Here's how the part is built. I have some questions about the finished solid (model axes, mm). Give positions to 0.01 mm unless a question says otherwise; leave off trailing zeros. Order: outer loops, then holes, each group sorted by start corner. A loop starts at its lowest first (then second) coordinate and runs counter-clockwise, first axis right, second up. Notation, with made-up numbers: M -31,-12.75 L -11,-12.75 A22 cw -11,25.25 Z; hole C -12.75,83 d7. An arc over 180 degrees is marked long. One line per item, written item: value. Start each with the question number.
from build123d import *

# Parameters (mm, degrees)
BOSS_EXTRUDE1_DEPTH = 3
FILLET1_R           = 4
FILLET2_R           = 3
FILLET3_R           = 1
FILLET4_R           = 0.5
SKETCH2_R           = 1
CUT_EXTRUDE1_DEPTH  = 2.3


with BuildPart() as part:
    # Sketch1 → Boss-Extrude1 (new body)
    with BuildSketch(Plane(origin=(0, 0, 0), x_dir=(1, 0, 0), z_dir=(0, 1, 0))):
        with BuildLine():
            Line((8.991433994, -0.392574486), (11.957374237, 67.538625463))
            ThreePointArc((11.957374237, 67.538625463), (7.303664413, 76.769797523), (-2.998880838, 77.623679297))
            Line((-2.998880838, 77.623679297), (-2.998880838, 43.087780912))
            Line((-2.998880838, 43.087780912), (-8.998880838, 39.623679297))
            Line((-8.998880838, 39.623679297), (-8.998880838, -0.141928385))
            ThreePointArc((-8.998880838, -0.141928385), (-0.125378351, -8.999126639), (8.991433994, -0.392574486))
        make_face()
    extrude(amount=BOSS_EXTRUDE1_DEPTH)

    # Fillet1
    fillet1_edges = [part.edges().sort_by_distance(p)[0] for p in [
        (-2.998880838, 1.5, -43.087780912),
    ]]
    fillet(fillet1_edges, radius=FILLET1_R)

    # Fillet2
    fillet2_edges = [part.edges().sort_by_distance(p)[0] for p in [
        (-2.998880838, 1.5, -77.623679297),
    ]]
    fillet(fillet2_edges, radius=FILLET2_R)

    # Fillet3
    fillet3_edges = [part.edges().sort_by_distance(p)[0] for p in [
        (-8.998880838, 1.5, -39.623679297),
    ]]
    fillet(fillet3_edges, radius=FILLET3_R)

    # Fillet4
    fillet4_edges = [part.edges().sort_by_distance(p)[0] for p in [
        (10.474404116, 3, -33.573025488),
        (-0.125378351, 3, 8.999126639),
        (-8.998880838, 3, -19.452200321),
        (-2.998880838, 3, -60.423029196),
        (-3.534779223, 3, -43.397181989),
        (8.325091375, 3, -75.986589378),
        (-2.306460594, 3, -77.365925089),
        (-6.748880838, 3, -40.922717403),
        (-8.864906242, 3, -39.546329028),
    ]]
    fillet(fillet4_edges, radius=FILLET4_R)

    # Sketch2 → Cut-Extrude1 (cut)
    with BuildSketch(Plane(origin=(0, 0, 0), x_dir=(-1, 0, 0), z_dir=(0, -1, 0))):
        with Locations((-6.916463595, 69.482266802)):
            Circle(SKETCH2_R)
        with Locations((-2.740849282, 1.610591965)):
            Circle(SKETCH2_R)
        with Locations((6, 35.355339106)):
            Circle(SKETCH2_R)
    extrude(amount=-CUT_EXTRUDE1_DEPTH, mode=Mode.SUBTRACT)


solid = part.part
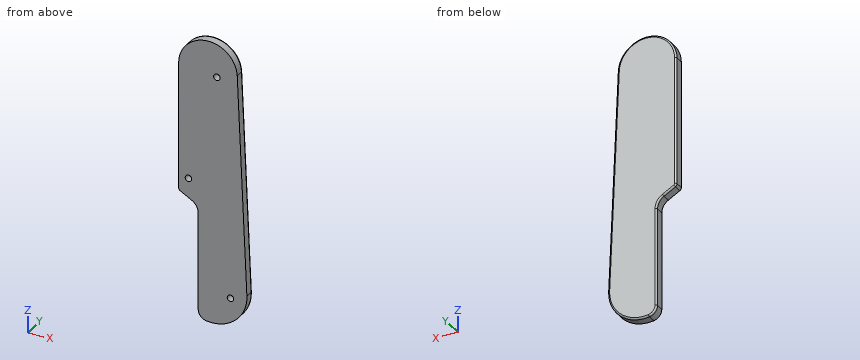
Item 1: I want a section at A-A on y = 0.95. Write out the boundary of the cut face in (x, z), plus the area to 3 significant figures.
Item 2: Will these pins go through, and if not, where does the flat tip stop? P1, Ø1.2, axis at x = -6, z = -35.36, coming from the -Y side; P2, Ø1, axis at y = 2, z = -10, coming from the +X side.
Item 3: Please list where these lines run through material, in increasing order: probe 1 along X at (y, z) = (0.45, -35); probe 2 along Z at (x, y) = (-6, 0.8); probe 3 along X at (y, z) = (0.6, -70). Write a range as [from, to].
Answer below:
1. outline: M -9,-39.05 A1 ccw -8.5,-39.91 L -5,-41.93 A4 cw -3,-45.4 L -3,-75.45 A3 ccw -0.55,-78.4 A10.58 ccw 11.96,-67.54 L 8.99,0.39 A9 ccw -9,0.14 Z; hole C -6,-35.36 d2; hole C 2.74,-1.61 d2; hole C 6.92,-69.48 d2
1. area: 1,420 mm²
2. P1: stops at y = 2.3
2. P2: stops at x = 9.47
3. probe 1: x = [-9, -6.93], [-5.07, 10.54]
3. probe 2: z = [-41.36, -36.36], [-34.36, 6.71]
3. probe 3: x = [-3, 6.06], [7.77, 11.78]
